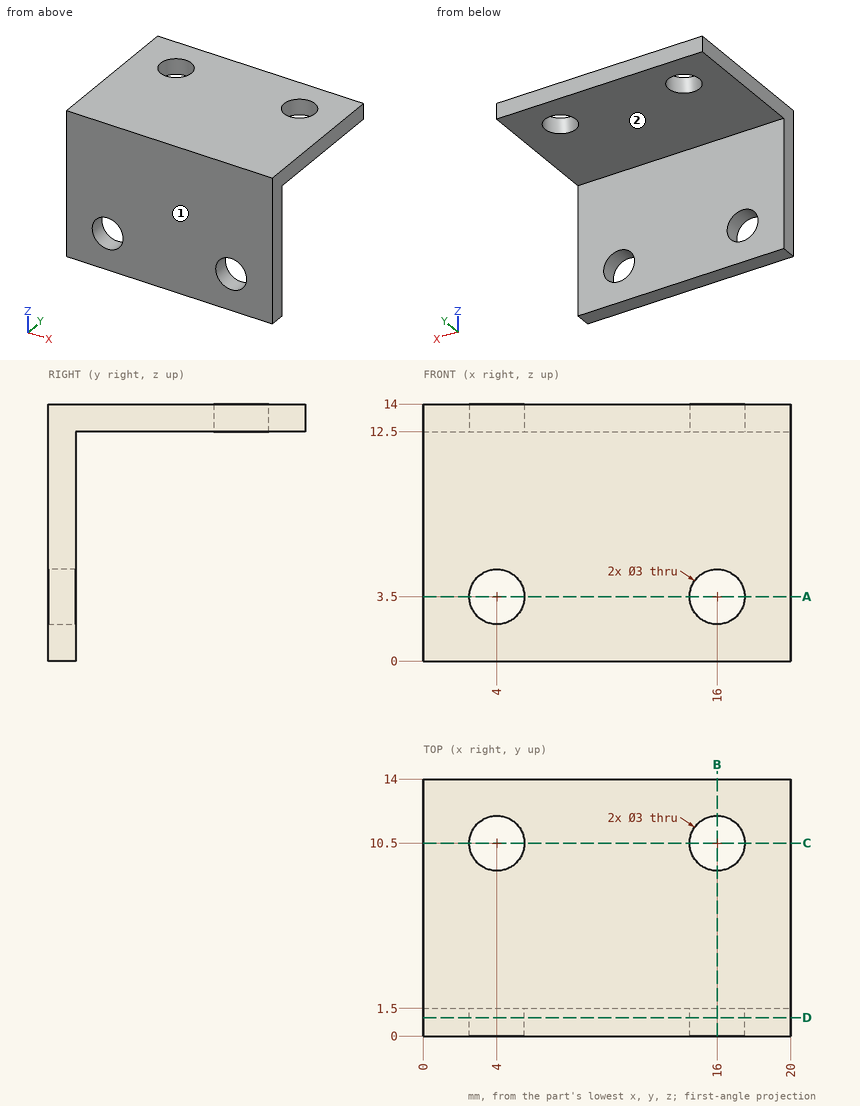
Study the drawing (mm; zero at the part's minimum x, y, z) and answer. A direction names the side the tool comes from. Coordinates: 2 decimals unless noted, no trailing zeros. Order: outer loops, then holes, each group sorted by start corner. A loop starts at its lowest first (then second) coordinate and runs counter-clockwise, first axis right, second up. Notation, with made-up numbers: M -30,-25.75 L 15,-25.75 A12 cw 15,-8.75 Z; hole C 68,22.25 d11. An arc over 180 degrees is marked long. Use CSV: the item, a comma, the result in double quotes.
Q1. Section C-C (y = 10.5) is taken. Determine the outline of the cut face in (x, z), then the cut area to 3 significant figures.
Here are the results:
outline,"M 0,12.5 L 2.5,12.5 L 2.5,14 L 0,14 Z; M 5.5,12.5 L 14.5,12.5 L 14.5,14 L 5.5,14 Z; M 17.5,12.5 L 20,12.5 L 20,14 L 17.5,14 Z"
area,"21.0 mm2"
Q2. Section A-A (z = 3.5) is taken. Determine the outline of the cut face in (x, y), then the cut area to 3 significant figures.
Here are the results:
outline,"M 0,0 L 2.5,0 L 2.5,1.5 L 0,1.5 Z; M 5.5,0 L 14.5,0 L 14.5,1.5 L 5.5,1.5 Z; M 17.5,0 L 20,0 L 20,1.5 L 17.5,1.5 Z"
area,"21.0 mm2"
Q3. Straight lines are drawn through the part: L1, parallel to X at y = 1.2, z = 3.5; L2, parallel to Y at x = 8, z = 5.75; L3, parallel to Z at x = 15.5, y = 9. For each, find the intervals that lie inside material, in ascending order.
Here are the results:
L1,"0 to 2.5, 5.5 to 14.5, 17.5 to 20"
L2,"0 to 1.5"
L3,"12.5 to 14"
Q4. Section D-D (y = 1) is taken. Determine the outline of the cut face in (x, z), then the cut area to 3 significant figures.
Here are the results:
outline,"M 0,0 L 20,0 L 20,14 L 0,14 Z; hole C 4,3.5 d3; hole C 16,3.5 d3"
area,"266 mm2"
Q5. A tool of negligible diameter and unlimited length cuts with its end or side. For the marked faces 1 and 2, from which of +Z, -Z, +X, -X, +Y, -Y can it reach the whole face along a straight path? Write none if from no direction.
Here are the results:
face 1,"+Z, -Z, +X, -X, -Y"
face 2,"-Z, +X, -X, +Y"
Q6. Given pin 1 Ø5 at (x, z) = (4, 3.5) entering from +Y; pin 2 Ø2.5 at (x, y) = (16, 10.5) entering from -Z, each flat-ended and moving along its own axis, determine where each tip first touches the part or whether it passes through.
Here are the results:
pin 1,"y = 1.5"
pin 2,"through"
Q7. Section B-B (x = 16) is taken. Determine the outline of the cut face in (y, z).
Here are the results:
outline,"M 0,0 L 1.5,0 L 1.5,2 L 0,2 Z; M 0,5 L 1.5,5 L 1.5,12.5 L 9,12.5 L 9,14 L 0,14 Z; M 12,12.5 L 14,12.5 L 14,14 L 12,14 Z"
